Geometry: final body of the model. Coordinates: model frame, mm. A direction names the side the tool comes from. Round coordinates to 2 decimals unless told otherwise and drop trailing zeros. Write each loop counter-clockwise with the first axis right and the second up, starting at its lowest first coordinate (ties: lowest second). Pieces come first, ordered by that corner, then holes.
Autodesk Inventor part; units mm, degrees
ref_plane "Start Plane" through (0, 0, 0) normal (0, 0, 1) x (1, 0, 0)
ref_plane "End Plane" through (0, 0, 360) normal (0, 0, 1) x (1, 0, 0)
ref_plane "YZ Plane" through (0, 0, 0) normal (1, 0, 0) x (0, 1, 0)
ref_plane "Start Plane" through (0, 0, 0) normal (0, 0, 1) x (1, 0, 0)
ref_plane "End Plane" through (0, 0, 360) normal (0, 0, 1) x (1, 0, 0)
sketch "Sketch" plane through (0, 0, 0) normal (0, 0, 1) x (1, 0, 0)
  line L0 (-10, -16) -> (-10, 16)
  line L1 (-6, 20) -> (6, 20)
  line L2 (10, 16) -> (10, -16)
  line L3 (6, -20) -> (-6, -20)
  arc A0 (-10, -16) -> (-6, -20) centre (-6, -16) ccw
  arc A1 (10, 16) -> (6, 20) centre (6, 16) ccw
  arc A2 (-6, 20) -> (-10, 16) centre (-6, 16) ccw
  arc A3 (6, -20) -> (10, -16) centre (6, -16) ccw
  arc A4 (-6, 18) -> (-8, 16) centre (-6, 16) ccw
  line L4 (-6, 18) -> (6, 18)
  arc A5 (8, 16) -> (6, 18) centre (6, 16) ccw
  line L5 (8, 16) -> (8, -16)
  arc A6 (6, -18) -> (8, -16) centre (6, -16) ccw
  line L6 (6, -18) -> (-6, -18)
  arc A7 (-8, -16) -> (-6, -18) centre (-6, -16) ccw
  line L7 (-8, -16) -> (-8, 16)
  line L8 (0, 29.1598) -> (0, -29.1598) construction
  line L9 (-15.1598, 0) -> (15.1598, 0) construction
  dimension "d7" = 4
  dimension "d9" = 20
  dimension "d11" = 40
  dimension "d12" = 2
  dimension "d15" = 10
  dimension "d16" = 20
extrude "Body" add sketch "Sketch" along normal up to surface (360 mm away) from surface at 0
sketch "Sketch3" plane through (0, 0, 0) normal (0, 0, 1) x (1, 0, 0)
  line L0 (0, 0) -> (10, 0)
ref_plane "Work Plane3" through (0, 0, 0) normal (0, -1, 0) x (1, 0, 0)
sketch "Sketch4" plane through (0, 0, 0) normal (0, -1, 0) x (1, 0, 0)
  line L0 (-2, 0) -> (12, 0)
  line L1 (-2, 360) -> (12, 360)
  dimension "d18" = 360
equation "\"d7\" = G_IR"
equation "\"d9\" = G_W"
equation "\"d11\" = G_H"
equation "\"d12\" = G_T"
equation "\"d15\" = 0.5 * d9"
equation "\"d16\" = 0.5 * d11"
equation "\"d3\" = G_L"
equation "\"G_W\" = 20"
equation "\"G_H\" = 40"
equation "\"G_T\" = 2"
equation "\"G_IR\" = 4"
equation "\"G_L\" = d18"
equation "\"G_OFFSET_START\" = 0"
properties part number "ISO 4019 - 40x20x2 - 360" material "Steel, Mild"
1) Draft query along X for faces 3 (the flat face through (10, 0, 177)), 4 (the flat face through (0, -18, 177)), 5 (the flat face through (-8.2, 0.1, 360)), 6 (the flat face through (-10, 0, 177)). Return one class per face: pulls with the +X half, pulls with the -X half, needs draft (parallel to the pull), parting line crosses it, or undercut.
2) Reachability of faces 1 (the flat face through (8, 0, 177)), 2 (the flat face through (-8.2, 0.1, 0)) from +Z, -Z, +X, -X, +Y, -Y: full face, straight path, thin tool, end or side. Return the list, or none.
3) Section A-A on y = 5.5. Output: boundary loops of the cut face in (x, z), plus the area to 3 significant figures.
4) Section B-B on z = 287.5. Output: boundary loops of the cut face in (x, y).
5) First-contact query: P1, Ø1, axis at x = 8, z = 297.5, coming from the -Y side; P2, Ø1.5, axis at x = -7, z = 113.5, coming from the -Y side. Flat tips, straight axial feed; report the tip coordinate or a pass-through.
6) Section C-C on x = 1.25. Output: boundary loops of the cut face in (y, z), plus the area to 3 significant figures.
7) Line query: probe 1 along Y at (x, z) = (0, 57.5); probe 2 along X at (y, z) = (5.5, 180.5); probe 3 along Y at (x, z) = (6.5, 277.5). Output: solid intervals per line, ascending.
Filled in:
1. face 3: pulls with the +X half
1. face 4: undercut
1. face 5: needs draft
1. face 6: pulls with the -X half
2. face 1: +Z, -Z
2. face 2: -Z, +X, -X, +Y, -Y
3. outline: (-10, 0) - (-8, 0) - (-8, 360) - (-10, 360) - close; (8, 0) - (10, 0) - (10, 360) - (8, 360) - close
3. area: 1,440 mm2
4. outline: (-10, -16) arc R4 ccw to (-6, -20) - (6, -20) arc R4 ccw to (10, -16) - (10, 16) arc R4 ccw to (6, 20) - (-6, 20) arc R4 ccw to (-10, 16) - close; hole (-8, -16) arc R2 ccw to (-6, -18) - (6, -18) arc R2 ccw to (8, -16) - (8, 16) arc R2 ccw to (6, 18) - (-6, 18) arc R2 ccw to (-8, 16) - close
5. P1: stops at y = -19.71
5. P2: stops at y = -19.99
6. outline: (-20, 0) - (-18, 0) - (-18, 360) - (-20, 360) - close; (18, 0) - (20, 0) - (20, 360) - (18, 360) - close
6. area: 1,440 mm2
7. probe 1: y = -20 to -18, 18 to 20
7. probe 2: x = -10 to -8, 8 to 10
7. probe 3: y = -19.97 to -17.94, 17.94 to 19.97
